Geometry check sheet. Reference: the model listing, model coordinates, mm. Face numbers are marked on the shaded views. A direction names the side the tool comes from. Give positions to 0.01 mm unless a question says otherwise; leave off trailing zeros. Loops run counter-clockwise (first coordinate to the right, second up) from the corner with the lowest first, then second, coordinate; pieces in that order, holes last. Notation, with made-up numbers: (-18, -25) -> (30, -25) arc R30 cw to (30, 5) -> close; hole circle Ø6 at (86.5, 69). An arc over 180 degrees is marked (long way). Answer as a JSON object with one key per item and string values.
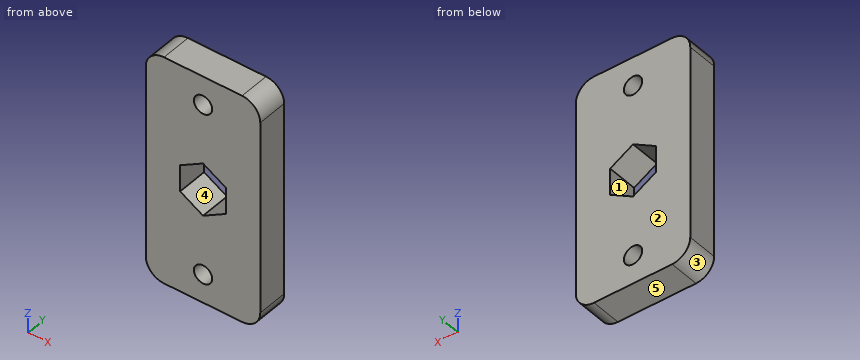
Autodesk Inventor part; units mm, degrees
ref_plane "YZ Plane" through (0, 0, 0) normal (1, 0, 0) x (0, 1, 0)
ref_plane "XZ Plane" through (0, 0, 0) normal (0, 1, 0) x (-1, 0, 0)
ref_plane "XY Plane" through (0, 0, 0) normal (0, 0, 1) x (1, 0, 0)
sketch "Sketch1" plane through (0, 0, 0) normal (0, 1, 0) x (-1, 0, 0)
  line L0 (10, 20) -> (-10, 20)
  line L1 (-10, 20) -> (-10, -20)
  line L2 (-10, -20) -> (10, -20)
  line L3 (10, -20) -> (10, 20)
  point P0 (0, 0)
  point P1 (10, 0)
  point P2 (0, 20)
  dimension "d0" = 20
  dimension "d1" = 40
extrude "Extrusion1" add sketch "Sketch1" along normal blind 5.334
sketch "Sketch2" plane through (0, 5.334, 0) normal (0, 1, 0) x (1, 0, 0)
  line L0 (0, 4.6188) -> (4, 2.3094)
  line L1 (4, 2.3094) -> (4, -2.3094)
  line L2 (4, -2.3094) -> (0, -4.6188)
  line L3 (0, -4.6188) -> (-4, -2.3094)
  line L4 (-4, -2.3094) -> (-4, 2.3094)
  line L5 (-4, 2.3094) -> (0, 4.6188)
  point P0 (0, 0)
  point P1 (0, 0)
  dimension "d4" = 8
extrude "Extrusion2" cut sketch "Sketch2" against normal through all
sketch "Sketch3" plane through (0, 5.334, 0) normal (0, 1, 0) x (1, 0, 0)
  point P0 (0, 0)
  point P1 (0, -15)
  point P2 (0, 15)
  dimension "d7" = 30
  dimension "d8" = 15
hole "Hole1" at (0, 5.334, 15) at (0, 5.334, -15) direction (0, -1, 0) diameter 3.2 end through all
fillet "Fillet1" radius 3.175 4 edges at (-10, 2.667, 20) (10, 2.667, 20) (10, 2.667, -20) (-10, 2.667, -20)
properties part number "hex_plate"
1) Section check A-A on z = 15. Record the cut outline in (x, y).
Geometry check:
{"outline": "(-10, 0) -> (-1.6, 0) -> (-1.6, 5.33) -> (-10, 5.33) -> close; (1.6, 0) -> (10, 0) -> (10, 5.33) -> (1.6, 5.33) -> close"}
2) Depth check by flat-ended pin: P1, Ø2.5, axis at x = 0, z = 15, coming from the +Y side. Enter the tip coordinate at first touch or a pass-through.
Geometry check:
{"P1": "passes through"}
3) Material ranges on line 1 along Z through (x, y) = (0, 1.7); line 2 along X through (y, z) = (3.15, 15); line 3 along Z through (x, y) = (0.75, 2.85), recorded low to high. Write a range as from..to.
Geometry check:
{"line 1": "z = -20..-16.6, -13.4..-4.62, 4.62..13.4, 16.6..20", "line 2": "x = -10..-1.6, 1.6..10", "line 3": "z = -20..-16.41, -13.59..-4.19, 4.19..13.59, 16.41..20"}
4) Section check B-B on y = 2.5. Record the cut outline in (x, z) (3 decimals), plus the area to 3 significant figures.
Geometry check:
{"outline": "(-10, -16.825) arc R3.175 ccw to (-6.825, -20) -> (6.825, -20) arc R3.175 ccw to (10, -16.825) -> (10, 16.825) arc R3.175 ccw to (6.825, 20) -> (-6.825, 20) arc R3.175 ccw to (-10, 16.825) -> close; hole (-4, -2.309) -> (0, -4.619) -> (4, -2.309) -> (4, 2.309) -> (0, 4.619) -> (-4, 2.309) -> close; hole circle Ø3.2 at (0, -15); hole circle Ø3.2 at (0, 15)", "area": "720 mm2"}
5) Draft check along X on the marked faces 3, 4 and 5. Enter one of: pulls with the +X half, pulls with the -X half, needs draft (parallel to the pull), parting line crosses it, or undercut.
Geometry check:
{"face 3": "pulls with the -X half", "face 4": "undercut", "face 5": "needs draft"}
6) Section check C-C on x = -0.5. Record the cut outline in (y, z), plus the area to 3 significant figures.
Geometry check:
{"outline": "(0, -20) -> (5.33, -20) -> (5.33, -16.52) -> (0, -16.52) -> close; (0, -13.48) -> (5.33, -13.48) -> (5.33, -4.33) -> (0, -4.33) -> close; (0, 4.33) -> (5.33, 4.33) -> (5.33, 13.48) -> (0, 13.48) -> close; (0, 16.52) -> (5.33, 16.52) -> (5.33, 20) -> (0, 20) -> close", "area": "135 mm2"}
7) Tool access check on the marked faces 1 and 2. Record the directions out of +Z, -Z, +X, -X, +Y, -Y that give a thin tool (end or side, any length) a straight path to the whole face; none if there is none.
Geometry check:
{"face 1": "+Y, -Y", "face 2": "+Z, -Z, +X, -X, +Y"}
8) Section check D-D on z = 4. Record the cut outline in (x, y), plus the area to 3 significant figures.
Geometry check:
{"outline": "(-10, 0) -> (-1.07, 0) -> (-1.07, 5.33) -> (-10, 5.33) -> close; (1.07, 0) -> (10, 0) -> (10, 5.33) -> (1.07, 5.33) -> close", "area": "95.2 mm2"}
